from build123d import *

# Parameters (mm, degrees)
SKETCH2_R          = 1.5
SKETCH2_R_2        = 1.7
BASE_FLANGE1_DEPTH = 5
FILLET1_R          = 15
FILLET2_R          = 10


# Sheet-metal steps are written as plain solids
with BuildPart() as part:
    # Sketch2 → Base-Flange1 (new body)
    with BuildSketch(Plane.XY):
        with BuildLine():
            Line((-6.5, 13), (6.5, 13))
            ThreePointArc((6.5, 13), (13.571067812, 10.071067812), (16.5, 3))
            Line((16.5, 3), (16.5, -38.5))
            Line((16.5, -38.5), (21.5, -38.5))
            Line((21.5, -38.5), (21.5, -43.5))
            Line((21.5, -43.5), (16.5, -43.5))
            Line((16.5, -43.5), (5, -43.5))
            Line((5, -43.5), (5, -47.5))
            Line((5, -47.5), (-5, -47.5))
            Line((-5, -47.5), (-5, -43.5))
            Line((-5, -43.5), (-28.5, -43.5))
            Line((-28.5, -43.5), (-28.5, -47.5))
            Line((-28.5, -47.5), (-38.5, -47.5))
            Line((-38.5, -47.5), (-38.5, -43.5))
            Line((-38.5, -43.5), (-73.5, -43.5))
            Line((-73.5, -43.5), (-73.5, -38.5))
            Line((-73.5, -38.5), (-38.5, -38.5))
            Line((-38.5, -38.5), (-38.5, -28.5))
            Line((-38.5, -28.5), (-16.5, -28.5))
            Line((-16.5, -28.5), (-16.5, 3))
            ThreePointArc((-16.5, 3), (-13.571067812, 10.071067812), (-6.5, 13))
        make_face()
        with Locations((-13.5, -6.5)):
            Circle(SKETCH2_R, mode=Mode.SUBTRACT)
        with Locations((-13.5, -30.5)):
            Circle(SKETCH2_R, mode=Mode.SUBTRACT)
        with Locations((13.5, -6.5)):
            Circle(SKETCH2_R, mode=Mode.SUBTRACT)
        with Locations((13.5, -30.5)):
            Circle(SKETCH2_R, mode=Mode.SUBTRACT)
        with Locations((19, -41)):
            Circle(SKETCH2_R_2, mode=Mode.SUBTRACT)
        with Locations((-71, -41)):
            Circle(SKETCH2_R_2, mode=Mode.SUBTRACT)
        with BuildLine():
            Line((-10, -5.678908346), (-10, -32.5))
            Line((-10, -32.5), (10, -32.5))
            Line((10, -32.5), (10, -5.678908346))
            ThreePointArc((10, -5.678908346), (0, 11.5), (-10, -5.678908346))
        make_face(mode=Mode.SUBTRACT)
    extrude(amount=-BASE_FLANGE1_DEPTH)

    # Fillet1
    # the kernel refuses this fillet: 15 mm, written as the material it adds along each edge
    with BuildSketch(Plane(origin=(-38.5, -38.5, 0), x_dir=(0, 1, 0), z_dir=(0, 0, -1))) as fillet1_piece_1:
        with BuildLine():
            CenterArc((15, -14.142135624), FILLET1_R, 109.471220634, 70.528779366)
            Line((0, -14.142135624), (-0.3, -14.142135624))
            Line((-0.3, -14.142135624), (-0.3, 0))
            Line((-0.3, 0), (0, 0.3))
            ThreePointArc((0, 0.3), (5, 0.3), (9.9, 0.282842712))
            Line((9.9, 0.282842712), (10, 0))
        make_face()
    extrude(amount=5)
    with BuildSketch(Plane(origin=(16.5, -38.5, 0), x_dir=(1, 0, 0), z_dir=(0, 0, -1))) as fillet1_piece_2:
        with BuildLine():
            CenterArc((15, -11.180339887), FILLET1_R, 131.810314896, 48.189685104)
            Line((0, -11.180339887), (-0.3, -11.180339887))
            Line((-0.3, -11.180339887), (-0.3, 0))
            Line((-0.3, 0), (0, 0.3))
            ThreePointArc((0, 0.3), (2.5, 0.3), (4.8, 0.223606798))
            Line((4.8, 0.223606798), (5, 0))
        make_face()
    extrude(amount=5)

    # Fillet2
    fillet2_edges = [part.edges().sort_by_distance(p)[0] for p in [
        (-38.5, -28.5, -2.5),
        (-16.5, -28.5, -2.5),
    ]]
    fillet(fillet2_edges, radius=FILLET2_R)


solid = part.part
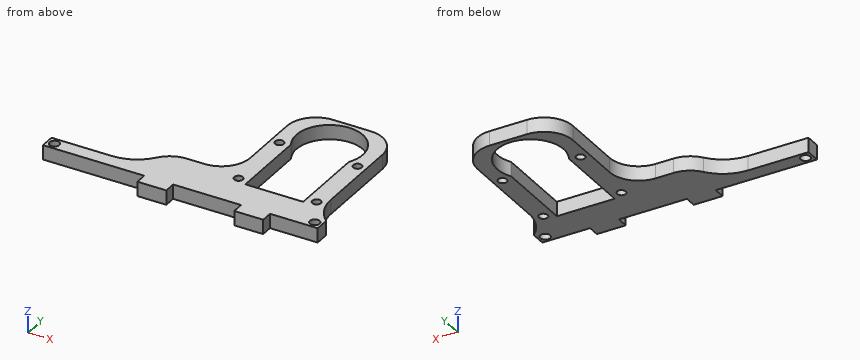
Model file for the job. Use its own axes, mm. Coordinates: 2 decimals unless noted, no trailing zeros. Loops run counter-clockwise (first coordinate to the right, second up) from the corner with the lowest first, then second, coordinate; pieces in that order, holes last. Notation, with made-up numbers: (26.5, 89.5) -> (41.5, 89.5) arc R20 cw to (41.5, 96.5) -> close; hole circle Ø1 at (33, 10). An arc over 180 degrees is marked (long way). Use one line per item in the form item = value. Start each with the question number.
(1) Cut at B-B on y = 0. Give the cut face in (x, z), and give its area (3 significant figures).
(2) Flat gauge pins, fed straight in: pin 1 (3 mm diameter, centred on y = -4.5, z = -2.5, fed in from +X); pin 2 (2.5 mm diameter, centred on y = -24.5, z = -2.5, fed in from -X); pin 3 (1.2 mm diameter, centred on y = -46.5, z = -2.5, fed in from -X). Where does each tip first touch, or does it go through?
(3) Cut at A-A on x = 0. Give the cut face in (y, z).
(4) Probe probe 1 along X at (y, z) = (-19, -3.65); probe 2 along X at (y, z) = (-31, -0.8); probe 3 along Y at (x, z) = (0, -2.3). List the from-to ranges inside material, lowest first. Write a range as from..to.
(5) Cut at D-D on z = -3.75. Give the number of separate pieces and of enclosed holes in the cut face, and give its area (3 significant figures).
(6) Cut at C-C on y = -41. Give the cut face in (x, z), and give its area (3 significant figures).
Values:
q1.outline = (-16.5, -5) -> (-11.5, -5) -> (-11.5, 0) -> (-16.5, 0) -> close; (11.5, -5) -> (16.5, -5) -> (16.5, 0) -> (11.5, 0) -> close
q1.area = 50.0 mm2
q2.pin_1 = 16.5
q2.pin_2 = -19.61
q2.pin_3 = -38.5
q3.outline = (-47.5, -5) -> (-32.5, -5) -> (-32.5, 0) -> (-47.5, 0) -> close; (11.5, -5) -> (13, -5) -> (13, 0) -> (11.5, 0) -> close
q4.probe_1 = -16.51..-10, 10..16.5
q4.probe_2 = -39.26..-14.91, -12.09..-10, 10..12.09, 14.91..16.96
q4.probe_3 = -47.5..-32.5, 11.5..13
q5.separate_pieces = 1
q5.enclosed_holes = 7
q5.area = 1,590 mm2
q6.outline = (-73.5, -5) -> (-72.7, -5) -> (-72.7, 0) -> (-73.5, 0) -> close; (-69.3, -5) -> (17.3, -5) -> (17.3, 0) -> (-69.3, 0) -> close; (20.7, -5) -> (21.5, -5) -> (21.5, 0) -> (20.7, 0) -> close
q6.area = 441 mm2
